from build123d import *

# Parameters (mm, degrees)
F1_DEPTH = 12.7
F3_DEPTH = 9.525
F5_D     = 6.604


# Not quite as in the source:
# - a pattern or mirror of a feature is missing from the dataset's text; its kind, count and spacing are read off the source's solid


with BuildPart() as f1:
    # F0 (on Front) → F1 (new body, symmetric)
    with BuildSketch(Plane.XZ):
        Polygon((-17.06248663, 1.7960512242), (-15.2664354058, 0), (15.2664354058, 0), (17.06248663, 1.7960512242), (1.27, 17.5885378542), (-1.27, 17.5885378542), align=None)
    extrude(amount=F1_DEPTH, both=True)

    # F2 (on Front) → F3 (cut, symmetric)
    with BuildSketch(Plane.XZ):
        Polygon((0, 11.6743329574), (-11.6743329574, 0), (11.6743329574, 0), align=None)
    extrude(amount=F3_DEPTH, both=True, mode=Mode.SUBTRACT)

    # F5 (through all)
    with Locations(Plane(origin=(5.8371664787, 0, 5.8371664787), x_dir=(0, -1, 0), z_dir=(-0.7071067812, 0, -0.7071067812))):
        with Locations((0, 0.635)):
            f5 = Hole(F5_D / 2)

    # F5_copies: F5 across plane
    add(f5.mirror(Plane(origin=(0, 0, 0), x_dir=(0, 0, -1), z_dir=(-1, 0, 0))), mode=Mode.SUBTRACT)


solid = f1.part
Geometry check sheet. Reference: the model listing, model coordinates, mm. A direction names the side the tool comes from. Round coordinates to 2 decimals unless told otherwise and drop trailing zeros. Loops run counter-clockwise (first coordinate to the right, second up) from the corner with the lowest first, then second, coordinate; pieces in that order, holes last. Notation, with made-up numbers: (-26.5, 59.5) - (-9.5, 59.5) arc R31 cw to (-9.5, 85.5) - close; hole circle Ø8 at (-7.75, 40). An arc over 180 degrees is marked (long way). Answer as CSV lines item,"result".
(1) Cross-section at B-B, the plane y = -2.75. Enter the section's corners in (x, z).
Output values:
outline,"(-17.06, 1.8) - (-15.27, 0) - (-11.67, 0) - (-6.68, 4.99) - (-10.27, 8.59) - close; (-7.69, 11.17) - (-4.1, 7.58) - (0, 11.67) - (4.1, 7.58) - (7.69, 11.17) - (1.27, 17.59) - (-1.27, 17.59) - close; (6.68, 4.99) - (11.67, 0) - (15.27, 0) - (17.06, 1.8) - (10.27, 8.59) - close"
(2) Cross-section at D-D, the plane y = -11. Enter the section's corners in (x, z).
Output values:
outline,"(-17.06, 1.8) - (-15.27, 0) - (15.27, 0) - (17.06, 1.8) - (1.27, 17.59) - (-1.27, 17.59) - close"
(3) Set-up check for faces 4 (the face through (0, 9.525, 5)), 5 (the face through (0, 11, 0)): record each of +Z, -Z, +X, -X, +Y, -Y from which the full face is reachable in a straight line by a thin tool's end or side.
Output values:
face 4,"-Z"
face 5,"-Z, +X, -X, +Y, -Y"
(4) Cross-section at A-A, the plane y = 4. Enter the section's corners in (x, z).
Output values:
outline,"(-17.06, 1.8) - (-15.27, 0) - (-11.67, 0) - (0, 11.67) - (11.67, 0) - (15.27, 0) - (17.06, 1.8) - (1.27, 17.59) - (-1.27, 17.59) - close"
(5) Cross-section at C-C, the plane x = -2. Enter the section's corners in (y, z) (3 decimals), and give its area (3 significant figures).
Output values:
outline,"(-12.7, 0) - (-9.525, 0) - (-9.525, 9.674) - (9.525, 9.674) - (9.525, 0) - (12.7, 0) - (12.7, 16.859) - (-12.7, 16.859) - close"
area,"244 mm²"
(6) Release check for a two-part mould opening along Z. For faces 1 (the face through (-7.3, 2.64, 11.56)), 2 (the face through (-5.241, 1.775, 10.076)), 3 (the face through (16.152, -0.178, 0.885)) record: released by +Z, released by -Z, zero draft, split by the parting line, or undercut.
Output values:
face 1,"released by +Z"
face 2,"undercut"
face 3,"released by -Z"
(7) Depth check by flat-ended pin: pin 1 Ø1 at (y, z) = (-9.5, 13.5) entering from +X; pin 2 Ø6 at (y, z) = (-9, 4) entering from -X; pin 3 Ø4 at (y, z) = (9, 14.5) entering from -X. Enter the tip coordinate at first touch or a pass-through.
Output values:
pin 1,"stops at x = 5.86"
pin 2,"stops at x = -17.06"
pin 3,"stops at x = -6.36"
(8) Material ranges on line 1 along Y through (x, z) = (-3, 4.75) (3 decimals); line 2 along X through (y, z) = (-7.75, 7); line 3 along X through (y, z) = (-4, 2.75), recorded low to high.
Output values:
line 1,"y = -12.7 to -9.525, 9.525 to 12.7"
line 2,"x = -11.86 to -4.67, 4.67 to 11.86"
line 3,"x = -16.11 to -8.92, 8.92 to 16.11"
